Source: CAD feature listing. Evaluate the final solid. Frame: model axes, mm. Give positions to 0.01 mm unless a question says otherwise; leave off trailing zeros. Loops run counter-clockwise (first coordinate to the right, second up) from the corner with the lowest first, then second, coordinate; pieces in that order, holes last.
```python
from build123d import *

# Parameters (mm, degrees)
BOSS_EXTRUDE1_DEPTH = 304.8
SKETCH3_W           = 2.5
SKETCH3_H           = 12.9625
CUT_EXTRUDE1_DEPTH  = 2.5875
SKETCH4_W           = 2.5
SKETCH4_H           = 50
CUT_EXTRUDE2_DEPTH  = 2.5875


with BuildPart() as part:
    # Sketch1 → Boss-Extrude1 (new body)
    with BuildSketch(Plane.XY):
        Polygon((0, 0), (0, 14.55), (1.5875, 14.55), (1.5875, 1.5875), (20.9125, 1.5875), (20.9125, 14.55), (22.5, 14.55), (22.5, 0), align=None)
    extrude(amount=BOSS_EXTRUDE1_DEPTH)

    # Sketch3 → Cut-Extrude1 (cut, through all)
    with BuildSketch(Plane.ZY.offset(-20.9125)):
        with Locations((293.55, 8.06875)):
            Rectangle(SKETCH3_W, SKETCH3_H)
    extrude(amount=-CUT_EXTRUDE1_DEPTH, mode=Mode.SUBTRACT)

    # Sketch4 → Cut-Extrude2 (cut, through all)
    with BuildSketch(Plane(origin=(0, 1.5875, 0), x_dir=(1, 0, 0), z_dir=(0, 1, 0))):
        with Locations((11.25, -25)):
            Rectangle(SKETCH4_W, SKETCH4_H)
    extrude(amount=-CUT_EXTRUDE2_DEPTH, mode=Mode.SUBTRACT)


solid = part.part
```
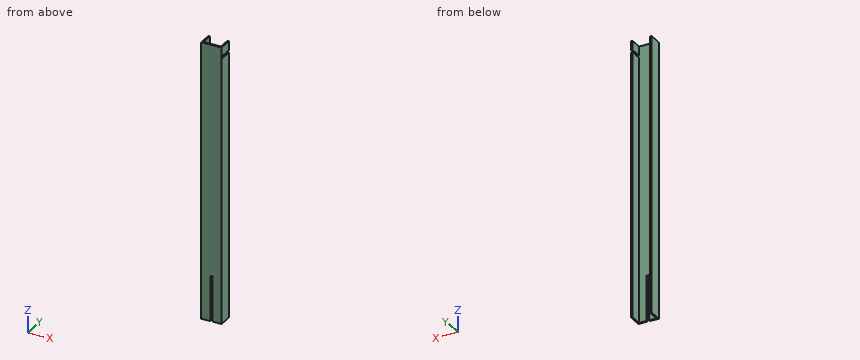
(1) Section B-B, the plane z = 273.5. Return the cut outline in (x, y), then the cut area to 3 significant figures.
A:
outline: (0, 0) - (22.5, 0) - (22.5, 14.55) - (20.91, 14.55) - (20.91, 1.59) - (1.59, 1.59) - (1.59, 14.55) - (0, 14.55) - close
area: 76.9 mm2
(2) Section A-A, the plane y = 12.25. Return the cut outline in (x, z).
A:
outline: (0, 0) - (1.59, 0) - (1.59, 304.8) - (0, 304.8) - close; (20.91, 0) - (22.5, 0) - (22.5, 292.3) - (20.91, 292.3) - close; (20.91, 294.8) - (22.5, 294.8) - (22.5, 304.8) - (20.91, 304.8) - close
(3) Section C-C, the plane x = 16.5. Return the cut outline in (y, z), then the cut area to 3 significant figures.
A:
outline: (0, 0) - (1.59, 0) - (1.59, 304.8) - (0, 304.8) - close
area: 484 mm2
(4) Ray query, line 1 along X through (y, z) = (9.5, 107); line 2 along Y through (x, z) = (2.5, 168). Return the intervals inside material, ascending.
A:
line 1: x = 0 to 1.59, 20.91 to 22.5
line 2: y = 0 to 1.59
(5) First-contact query: pin 1 (3 mm diameter, centred on x = 6, z = 272, fed in from +Y); pin 2 (0.5 mm diameter, centred on x = 11, y = 0.5, fed in from -Z). Flat tips, straight axial feed; report the tip coordinate or a pass-through.
A:
pin 1: stops at y = 1.59
pin 2: stops at z = 50
